from build123d import *

# Parameters (mm, degrees)
EXTRUDE_THIN1_DEPTH = 11.43
SKETCH2_R           = 3.96875
CUT_EXTRUDE1_DEPTH  = 87.407822566
SKETCH3_W           = 127
SKETCH3_H           = 76.2
CUT_EXTRUDE2_DEPTH  = 6.35


with BuildPart() as part:
    # Sketch1 → Extrude-Thin1 (new body)
    with BuildSketch(Plane(origin=(0, 0, 0), x_dir=(1, 0, 0), z_dir=(0, 1, 0))):
        with BuildLine():
            Line((-36.661742094, -61.2775), (36.661742094, -61.2775))
            ThreePointArc((36.661742094, -61.2775), (56.73404589, -49.68875), (56.73404589, -26.51125))
            Line((56.73404589, -26.51125), (20.072303796, 36.98875))
            ThreePointArc((20.072303796, 36.98875), (0, 48.5775), (-20.072303796, 36.98875))
            Line((-20.072303796, 36.98875), (-56.73404589, -26.51125))
            ThreePointArc((-56.73404589, -26.51125), (-56.73404589, -49.68875), (-36.661742094, -61.2775))
        make_face()
        with BuildLine():
            Line((-36.661742094, -40.3225), (36.661742094, -40.3225))
            ThreePointArc((36.661742094, -40.3225), (38.586483553, -39.21125), (38.586483553, -36.98875))
            Line((38.586483553, -36.98875), (1.92474146, 26.51125))
            ThreePointArc((1.92474146, 26.51125), (0, 27.6225), (-1.92474146, 26.51125))
            Line((-1.92474146, 26.51125), (-38.586483553, -36.98875))
            ThreePointArc((-38.586483553, -36.98875), (-38.586483553, -39.21125), (-36.661742094, -40.3225))
        make_face(mode=Mode.SUBTRACT)
    extrude(amount=EXTRUDE_THIN1_DEPTH)

    # Sketch2 → Cut-Extrude1 (cut, through all)
    with BuildSketch(Plane(origin=(0, 0, 0), x_dir=(1, 0, 0), z_dir=(0, 1, 0))):
        with Locations(Location((-50.409895379, -46.0375, 0), (0, 0, 270))):
            Circle(SKETCH2_R)
        with Locations(Location((0, 41.275, 0), (0, 0, 270))):
            Circle(SKETCH2_R)
        with Locations(Location((50.409895379, -46.0375, 0), (0, 0, 270))):
            Circle(SKETCH2_R)
    extrude(amount=CUT_EXTRUDE1_DEPTH, mode=Mode.SUBTRACT)

    # Sketch3 → Cut-Extrude2 (cut)
    with BuildSketch(Plane(origin=(0, 0, 0), x_dir=(1, 0, 0), z_dir=(0, 1, 0))):
        with Locations((0, 22.86)):
            Rectangle(SKETCH3_W, SKETCH3_H)
    extrude(amount=CUT_EXTRUDE2_DEPTH, mode=Mode.SUBTRACT)


solid = part.part
Source: CAD feature listing. Evaluate the final solid. Frame: model axes, mm. A direction names the side the tool comes from. Round coordinates to 2 decimals unless told otherwise and drop trailing zeros. Loops run counter-clockwise (first coordinate to the right, second up) from the corner with the lowest first, then second, coordinate; pieces in that order, holes last.
Q1. Access query for faces 1 (the face through (-38, 3, 15.24)), 2 (the face through (-56.9, 5.6, 49.4)), 3 (the face through (38.57, 5.63, 39.24)). Directions: +Z, -Z, +X, -X, +Y, -Y. A direction counts if a zero-diameter tool reaches every point of the face in a straight line with its end or side. Return the directions, or none.
Q2. First-contact query: P1, Ø4, axis at x = 42.5, z = 45.5, coming from the -Y side; P2, Ø4, axis at y = 9, z = 30, coming from the -X side; P3, Ø1.5, axis at x = -28.5, y = 9.5, coming from the -Z side; P4, Ø2, axis at y = 7, z = 10.5, coming from the +X side. Flat tips, straight axial feed; report the tip coordinate or a pass-through.
Q3. Ray query, line 1 (Z direction, x = 0, y = 8.85); line 2 (X direction, y = 4.25, z = 43); line 3 (Z direction, x = 49, y = 6). Return the intervals inside material, ascending.
Q4. Section A-A, the plane x = 0. Return loops of the section in (y, z).
Q5. Mould query, pull axis X, two halves, no side actions, for faces 4 (the face through (0.033, 8.854, -27.622)), 5 (the face through (-42.22, 8.17, 1.37)), 6 (the face through (-1, 11.43, 42)), 7 (the face through (-24.073, 6.905, 11.85)). Classes: pulls with the +X half, pulls with the -X half, needs draft (parallel to the pull), parting line crosses it, or undercut.
Q6. Section B-B, the plane y = 3.5. Return loops of the section in (x, z) (1 decimal), plus the area to 3 significant figures.
Q7. Section C-C, the plane z = 1.5. Return loops of the section in (x, y), plus the area to 3 significant figures.
Solutions:
1. face 1: -Z, +X, -X, -Y
1. face 2: -X, +Y, -Y
1. face 3: +Y, -Y
2. P1: stops at y = 0
2. P2: stops at x = -59.02
2. P3: stops at z = -23.69
2. P4: stops at x = 48.07
3. line 1: z = -48.58 to -45.24, -37.31 to -27.62, 40.32 to 61.28
3. line 2: x = -59.32 to -52.96, -47.86 to 47.86, 52.96 to 59.32
3. line 3: z = 15.24 to 42.33, 49.75 to 57.72
4. outline: (0, 40.32) - (11.43, 40.32) - (11.43, 61.28) - (0, 61.28) - close; (6.35, -48.58) - (11.43, -48.58) - (11.43, -45.24) - (6.35, -45.24) - close; (6.35, -37.31) - (11.43, -37.31) - (11.43, -27.62) - (6.35, -27.62) - close
5. face 4: undercut
5. face 5: pulls with the -X half
5. face 6: needs draft
5. face 7: undercut
6. outline: (-56.7, 26.5) - (-50.2, 15.2) - (-26, 15.2) - (-38.6, 37) arc R2.2 cw to (-36.7, 40.3) - (36.7, 40.3) arc R2.2 cw to (38.6, 37) - (26, 15.2) - (50.2, 15.2) - (56.7, 26.5) arc R23.2 ccw to (36.7, 61.3) - (-36.7, 61.3) arc R23.2 ccw to start; hole circle Ø7.9 at (-50.4, 46); hole circle Ø7.9 at (50.4, 46)
6. area: 3,350 mm2
7. outline: (-42.29, 6.35) - (-18.1, 6.35) - (-18.1, 11.43) - (-42.29, 11.43) - close; (18.1, 6.35) - (42.29, 6.35) - (42.29, 11.43) - (18.1, 11.43) - close
7. area: 246 mm2
